```python
from build123d import *

# Parameters (mm, degrees)
SKETCH1_R           = 6
SKETCH1_R_2         = 1.5
SKETCH1_W           = 8
SKETCH1_H           = 2.4
BOSS_EXTRUDE1_DEPTH = 5
SKETCH2_R           = 1.2
CUT_EXTRUDE1_DEPTH  = 6


with BuildPart() as part:
    # Sketch1 → Boss-Extrude1 (new body)
    with BuildSketch(Plane(origin=(0, 0, 0), x_dir=(0, 0, -1), z_dir=(1, 0, 0))):
        Polygon((0, 0), (-50, 0), (-50, 25), (-55, 25), (-55, 40), (-50, 40), (-50, 47), (-45, 47), (-45, 53), (-50, 53), (-50, 64), (0, 64), (0, 49), (-5, 49), (-5, 24), (0, 24), align=None)
        with Locations((-20, 17)):
            Circle(SKETCH1_R, mode=Mode.SUBTRACT)
        with Locations((-45, 7.5)):
            Circle(SKETCH1_R_2, mode=Mode.SUBTRACT)
        with Locations((-32, 7.5)):
            Circle(SKETCH1_R_2, mode=Mode.SUBTRACT)
        with Locations((-38.5, 18.2)):
            Rectangle(SKETCH1_W, SKETCH1_H, mode=Mode.SUBTRACT)
    extrude(amount=BOSS_EXTRUDE1_DEPTH)

    # Sketch2 → Cut-Extrude1 (cut, through all)
    with BuildSketch(Plane(origin=(5, 0, 0), x_dir=(0, 0, -1), z_dir=(1, 0, 0))):
        with Locations((-2.5, 56.5)):
            Circle(SKETCH2_R)
        with Locations((-2.5, 12)):
            Circle(SKETCH2_R)
        Polygon((-50, 59.7), (-46, 59.7), (-46, 61.25), (-44.2, 61.25), (-44.2, 59.7), (-42.2, 59.7), (-42.2, 57.3), (-44.2, 57.3), (-44.2, 55.75), (-46, 55.75), (-46, 57.3), (-50, 57.3), align=None)
        Polygon((-44.2, 19.4), (-42.2, 19.4), (-42.2, 17), (-44.2, 17), (-44.2, 15.45), (-46, 15.45), (-46, 17), (-50, 17), (-50, 19.4), (-46, 19.4), (-46, 20.95), (-44.2, 20.95), align=None)
    extrude(amount=-CUT_EXTRUDE1_DEPTH, mode=Mode.SUBTRACT)


solid = part.part
```
Design review of the part built by this model. Coordinates are the model's own, in mm. A direction names the side the tool comes from. Coordinates: 2 decimals unless noted, no trailing zeros. Loops run counter-clockwise (first coordinate to the right, second up) from the corner with the lowest first, then second, coordinate; pieces in that order, holes last.
Q1. We need section C-C on y = 56.5. State the section outline as (x, z) points, and give its area (3 significant figures).
Reported:
outline: (0, 0) - (5, 0) - (5, 1.3) - (0, 1.3) - close; (0, 3.7) - (5, 3.7) - (5, 44.2) - (0, 44.2) - close; (0, 46) - (5, 46) - (5, 50) - (0, 50) - close
area: 229 mm2
Q2. We need section D-D on z = 20. State the section outline as (x, y) points, and give its area (3 significant figures).
Reported:
outline: (0, 0) - (5, 0) - (5, 11) - (0, 11) - close; (0, 23) - (5, 23) - (5, 64) - (0, 64) - close
area: 260 mm2
Q3. For pin 1 (2.5 mm diameter, centred on y = 7.5, z = 45, fed in from -X) (1 decimal); pin 2 (1.5 mm diameter, centred on x = 2, y = 51, fed in from +Z); pin 3 (1.7 mm diameter, centred on x = 2, y = 20, fed in from +Z); pin 4 (2.5 mm diameter, centred on x = 1.5, z = 53, fed in from -Y), all flat-tipped, find the tip position at first contact; note any pin that passes through.
Reported:
pin 1: passes through
pin 2: stops at z = 45
pin 3: stops at z = 50
pin 4: stops at y = 25
Q4. Tool access review of faces 1 (the face through (0, 32, 27)), 2 (the face through (3, 60, 44.2)), 3 (the face through (2, 37, 5)), 4 (the face through (2, 17, 39)): name each direction out of +Z, -Z, +X, -X, +Y, -Y from which nothing blocks a thin tool from reaching the whole face with its end or side.
Reported:
face 1: +Z, -Z, -X, +Y, -Y
face 2: +X, -X
face 3: -Z, +X, -X
face 4: +Z, +X, -X
Q5. We need section B-B on z = 2.5. State the section outline as (x, y) points, and give its area (3 significant figures).
Reported:
outline: (0, 0) - (5, 0) - (5, 10.8) - (0, 10.8) - close; (0, 13.2) - (5, 13.2) - (5, 24) - (0, 24) - close; (0, 49) - (5, 49) - (5, 55.3) - (0, 55.3) - close; (0, 57.7) - (5, 57.7) - (5, 64) - (0, 64) - close
area: 171 mm2
Q6. The part is to be moulded in two halves that separate along Z. For faces 5 (the face through (2, 50, 45)), 6 (the face through (3, 20.95, 45)), 7 (the face through (2, 0, 25)), say which applies: +Z half, -Z half, draft (parallel to the pull), parting line (faces both ways), or undercut.
Reported:
face 5: +Z half
face 6: undercut
face 7: draft
Q7. We need section A-A on z = 32. State the section outline as (x, y) points, and give its area (3 significant figures).
Reported:
outline: (0, 0) - (5, 0) - (5, 6) - (0, 6) - close; (0, 9) - (5, 9) - (5, 64) - (0, 64) - close
area: 305 mm2
Q8. To check wall thickness, follow line 1 (Y direction, x = 0.7, z = 45.5); line 2 (Y direction, x = 3.8, z = 2.5); line 3 (Y direction, x = 3.6, z = 42). State the ranges of each line that lie inside material, in increasing order.
Reported:
line 1: y = 0 to 6.09, 8.91 to 15.45, 20.95 to 47, 53 to 55.75, 61.25 to 64
line 2: y = 0 to 10.8, 13.2 to 24, 49 to 55.3, 57.7 to 64
line 3: y = 0 to 17, 19.4 to 64
